Part model, mm, in its own coordinate system. Face numbers are marked on the shaded views. Coordinates: 2 decimals unless noted, no trailing zeros. Order: outer loops, then holes, each group sorted by start corner. A loop starts at its lowest first (then second) coordinate and runs counter-clockwise, first axis right, second up. Notation, with made-up numbers: (7.5, 0.25) - (23.5, 0.25) arc R23 ccw to (23.5, 16.25) - close; hole circle Ø7 at (41.25, -20). An arc over 180 degrees is marked (long way). Use a Markdown table: item, result. Add a question column.
1) Drop flat-ended pins along their axis: P1, Ø3, axis at y = -84, z = -32, coming from the +X side; P2, Ø8, axis at x = 50.5, y = -53, coming from the -Z side; P3, Ø5, axis at y = -59.5, z = -48.5, coming from the -X side. Give the stop position or say it passes through.
2) Saw through at A-A on y = -54. List the corners of the cut face in (x, z).
3) Saw through at B-B on z = -71. List the corners of the cut face in (x, y), then the cut area to 3 significant figures.
4) Two-plate mould, pull along Z, no slides. Class the marked faces 1, 2 and 3: +Z half, -Z half, draft (parallel to the pull), parting line (faces both ways), or undercut.
5) Wall check: L1, parallel to X at y = -92.5, z = -26; L2, parallel to Z at x = 25, y = -75.5; L3, parallel to Z at x = 23, y = -12.5. Give the ranges that are in metal, low to high. Write a range as [from, to].
6) Saw through at C-C on x = 7. List the corners of the cut face in (y, z).
```python
from build123d import *

# Parameters (mm, degrees)
F1_DEPTH = 127


with BuildPart() as f1:
    # F0 (on Front) → F1 (new body)
    with BuildSketch(Plane.XZ):
        Polygon((58.567305, -33.813849), (0, -67.627698), (-12.155358, -60.609799), (17.128294, -91.552522), (58.567305, -81.663497), (70.722663, -40.831748), (58.567305, -27.987726), align=None)
        Polygon((-12.155358, -60.609799), (0, -67.627698), (58.567305, -33.813849), (58.567305, -27.987726), (41.43901, -9.889025), (0, -19.778051), align=None)
    extrude(amount=F1_DEPTH)


solid = f1.part
```
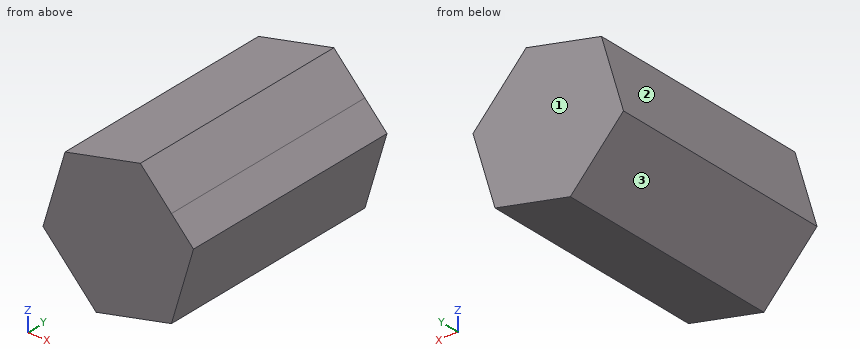
Results are:
| question | item | result |
|---|---|---|
| 1 | P1 | x = 63.78 |
| 1 | P2 | z = -84.54 |
| 1 | P3 | x = -9.29 |
| 2 | outline | (-12.16, -60.61) - (17.13, -91.55) - (58.57, -81.66) - (70.72, -40.83) - (41.44, -9.89) - (0, -19.78) - close |
| 3 | outline | (-2.32, -127) - (61.74, -127) - (61.74, 0) - (-2.32, 0) - close |
| 3 | area | 8,140 mm2 |
| 4 | face 1 | draft |
| 4 | face 2 | +Z half |
| 4 | face 3 | -Z half |
| 5 | L1 | [-1.85, 56.69] |
| 5 | L2 | [-89.67, -13.81] |
| 5 | L3 | [-90.15, -14.29] |
| 6 | outline | (-127, -80.85) - (0, -80.85) - (0, -18.11) - (-127, -18.11) - close |
